Model file for the job. Use its own axes, mm. Face numbers are marked on the shaded views. A direction names the side the tool comes from. Round coordinates to 2 decimals unless told otherwise and drop trailing zeros. Write each loop counter-clockwise with the first axis right and the second up, starting at its lowest first coordinate (ties: lowest second). Pieces come first, ordered by that corner, then holes. Notation, with made-up numbers: (-37, 75.25) - (17, 75.25) arc R24 cw to (17, 89.25) - close; hole circle Ø1 at (-25.75, 28.25). An arc over 180 degrees is marked (long way). Answer as a JSON object with one key per item and string values. Group by question number.
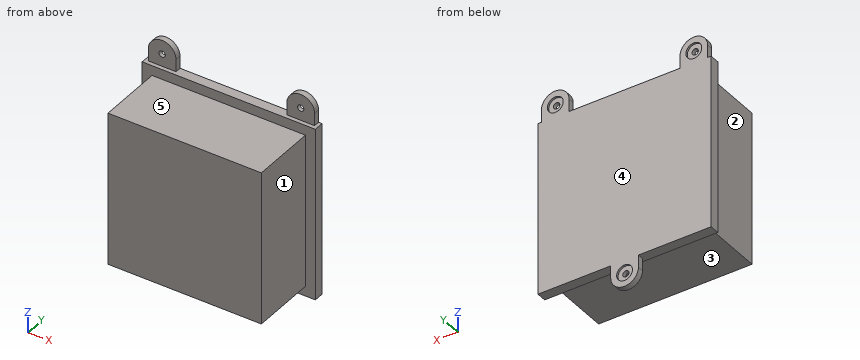
from build123d import *

# Parameters (mm, degrees)
F1_DEPTH       = 3
F2_D           = 3.2
F2_CBORE_D     = 8
F2_CBORE_DEPTH = 1
F4_DEPTH       = 2
F5_W           = 77.5
F5_H           = 77.5
F6_DEPTH       = 33


with BuildPart() as f1:
    # F0 (on Front) → F1 (new body)
    with BuildSketch(Plane.XZ):
        with BuildLine():
            Line((-31.8941220641, 46.416635698), (-31.8941220641, -41.083364302))
            Line((-31.8941220641, -41.083364302), (4.8558779359, -41.083364302))
            Line((4.8558779359, -41.083364302), (4.8558779359, -47.333364302))
            ThreePointArc((4.8558779359, -47.333364302), (11.8558779359, -54.333364302), (18.8558779359, -47.333364302))
            Line((18.8558779359, -47.333364302), (18.8558779359, -41.083364302))
            Line((18.8558779359, -41.083364302), (55.6058779359, -41.083364302))
            Line((55.6058779359, -41.083364302), (55.6058779359, 46.416635698))
            Line((55.6058779359, 46.416635698), (53.8558779359, 46.416635698))
            Line((53.8558779359, 46.416635698), (53.8558779359, 52.666635698))
            ThreePointArc((53.8558779359, 52.666635698), (46.8558779359, 59.666635698), (39.8558779359, 52.666635698))
            Line((39.8558779359, 52.666635698), (39.8558779359, 46.416635698))
            Line((39.8558779359, 46.416635698), (-16.1441220641, 46.416635698))
            Line((-16.1441220641, 46.416635698), (-16.1441220641, 52.666635698))
            ThreePointArc((-16.1441220641, 52.666635698), (-23.1441220641, 59.666635698), (-30.1441220641, 52.666635698))
            Line((-30.1441220641, 52.666635698), (-30.1441220641, 46.416635698))
            Line((-30.1441220641, 46.416635698), (-31.8941220641, 46.416635698))
        make_face()
    extrude(amount=F1_DEPTH)

    # F2 (through all)
    with Locations(Plane(origin=(0, 0, 0), x_dir=(1, 0, 0), z_dir=(0, 1, 0))):
        with Locations((-23.1441220641, -52.666635698), (46.8558779359, -52.666635698), (11.8558779359, 47.333364302)):
            CounterBoreHole(F2_D / 2, F2_CBORE_D / 2, F2_CBORE_DEPTH)

    # F3 (on face) → F4 (join)
    with BuildSketch(Plane.XZ.offset(3)):
        Polygon((-30.1441220641, 46.416635698), (-31.8941220641, 46.416635698), (-31.8941220641, -41.083364302), (4.8558779359, -41.083364302), (18.8558779359, -41.083364302), (55.6058779359, -41.083364302), (55.6058779359, 46.416635698), (53.8558779359, 46.416635698), (39.8558779359, 46.416635698), (-16.1441220641, 46.416635698), align=None)
    extrude(amount=F4_DEPTH)

    # F5 (on face) → F6 (join)
    with BuildSketch(Plane.XZ.offset(5)):
        with Locations((11.8558779359, 2.666635698)):
            Rectangle(F5_W, F5_H)
    extrude(amount=F6_DEPTH)


solid = f1.part
(1) Slice it at D-D (y = -7). Write the cut outline in (x, z), then the cut area to 3 significant figures.
(2) Slice it at C-C (x = -14). Write the cut outline in (y, z).
(3) 3-axis set-ups, long thin cutter, end or side, ignore diameter. For the marked faces 1, 2, 3, 4 and 5: which of +Z, -Z, +X, -X, +Y, -Y reach the whole face in a straight line?
(4) Flat gauge pins, fed straight in: pin 1 (3.5 mm diameter, centred on y = -1.5, z = 48.5, fed in from -X); pin 2 (5.5 mm diameter, centred on x = -3, y = -2, fed in from -Z); pin 3 (8 mm diameter, centred on x = 26, y = -13, fed in from +Z). Where does each tip first touch, or does it go through?
(5) Slice it at B-B (x = 11.5). Write the cut outline in (y, z).
(6) Drill centre lines: line 1 (X direction, y = -6, z = -11.5); line 2 (Z direction, x = 9, y = -18.5); line 3 (Y direction, x = -7.5, z = 41.5). Where is each one in solid material? Low to high. Write a range as from..to.
(7) Slice it at A-A (z = 18.5). Write the cut outline in (x, y).
Answer:
{
 "1": {"outline": "(-26.89, -36.08) - (50.61, -36.08) - (50.61, 41.42) - (-26.89, 41.42) - close", "area": "6,010 mm²"},
 "2": {"outline": "(-38, -36.08) - (-5, -36.08) - (-5, -41.08) - (0, -41.08) - (0, 46.42) - (-5, 46.42) - (-5, 41.42) - (-38, 41.42) - close"},
 "3": {"face 1": "+Z, -Z, +X, -Y", "face 2": "+Z, -Z, -X, -Y", "face 3": "-Z, +X, -X, -Y", "face 4": "+Z, -Z, +X, -X, +Y", "face 5": "+Z, +X, -X, -Y"},
 "4": {"pin 1": "x = -30.14", "pin 2": "z = -41.08", "pin 3": "z = 41.42"},
 "5": {"outline": "(-38, -36.08) - (-5, -36.08) - (-5, -41.08) - (-3, -41.08) - (-3, -45.77) - (-1, -45.77) - (-1, -43.35) - (0, -43.35) - (0, 46.42) - (-5, 46.42) - (-5, 41.42) - (-38, 41.42) - close; (-3, -54.32) - (0, -54.32) - (0, -51.32) - (-1, -51.32) - (-1, -48.89) - (-3, -48.89) - close"},
 "6": {"line 1": "-26.89..50.61", "line 2": "-36.08..41.42", "line 3": "-5..0"},
 "7": {"outline": "(-31.89, -5) - (-26.89, -5) - (-26.89, -38) - (50.61, -38) - (50.61, -5) - (55.61, -5) - (55.61, 0) - (-31.89, 0) - close"}
}
